Here's how the part is built. I have some questions about the finished solid (model axes, mm). Round coordinates to 2 decimals unless told otherwise and drop trailing zeros. Order: outer loops, then holes, each group sorted by start corner. A loop starts at its lowest first (then second) coordinate and runs counter-clockwise, first axis right, second up. Notation, with made-up numbers: (-5, 31) - (29, 31) arc R28 cw to (29, 67) - close; hole circle Ø10 at (75, -23). An arc over 180 degrees is marked (long way). One line per item, written item: value.
from build123d import *

# Parameters (mm, degrees)
F1_DEPTH = 85
F2_W     = 3.5
F2_H     = 3.5
F3_DEPTH = 3.5
F4_W     = 3.5
F4_H     = 3.5
F5_DEPTH = 3.5


with BuildPart() as f1:
    # F0 (on Top) → F1 (new body)
    with BuildSketch(Plane.XY):
        Polygon((-25, -42.409548), (-25, -34.409548), (-32.608452, -36.881684), (-30.81234, -42.409548), align=None)
    extrude(amount=F1_DEPTH)

    # F2 (on face) → F3 (cut)
    with BuildSketch(Plane.YZ.offset(-25)):
        with Locations((-37.659548, 6.25)):
            Rectangle(F2_W, F2_H)
        with Locations((-37.659548, 28.25)):
            Rectangle(F2_W, F2_H)
    extrude(amount=-F3_DEPTH, mode=Mode.SUBTRACT)

    # F4 (on face) → F5 (cut)
    with BuildSketch(Plane(origin=(7.725425, -23.776413, 0), x_dir=(-0.951057, -0.309017, 0), z_dir=(-0.309017, 0.951057, 0))):
        with Locations((37.659548, 6.25)):
            Rectangle(F4_W, F4_H)
        with Locations((37.659548, 28.25)):
            Rectangle(F4_W, F4_H)
    extrude(amount=-F5_DEPTH, mode=Mode.SUBTRACT)


solid = f1.part
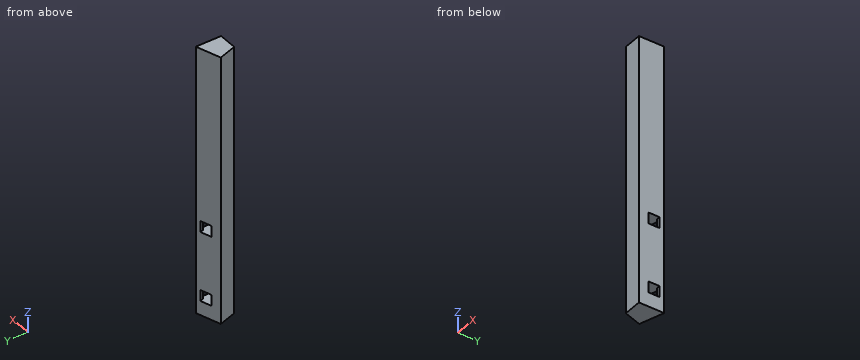
Q1. If I drill on line 1 along Z through (x, y) = (-27.75, -36.5); line 2 along Y through (x, z) = (-25.5, 72); line 3 along Y through (x, z) = (-26, 38.5), over which ranges is the centre line in solid material (lowest first)?
Results list:
line 1: 0 to 4.5, 8 to 26.5, 30 to 85
line 2: -42.41 to -34.57
line 3: -42.41 to -34.73
Q2. Will these pins go through, and if not, where does the flat tip stop? pin 1 (1 mm diameter, centred on x = -26.5, z = 28, fed in from +Y); pin 2 (2 mm diameter, centred on y = -38.5, z = 29.5, fed in from -X); pin 3 (1.5 mm diameter, centred on x = -29, z = 19, fed in from +Y).
Results list:
pin 1: y = -34.73
pin 2: x = -32.41
pin 3: y = -35.47
Q3. If we section it at A-A, the plane y = -38.5: Please give me the cut outline in (x, z).
Results list:
outline: (-32.08, 0) - (-25, 0) - (-25, 4.5) - (-28.93, 4.5) - (-28.93, 8) - (-25, 8) - (-25, 26.5) - (-28.93, 26.5) - (-28.93, 30) - (-25, 30) - (-25, 85) - (-32.08, 85) - close
Q4. If we section it at C-C, the plane x = -31.75: Please give me the cut outline in (y, z).
Results list:
outline: (-39.52, 0) - (-36.6, 0) - (-36.6, 85) - (-39.52, 85) - close
Q5. If we section it at B-B, the plane z = 69.5: Please give me the cut outline in (x, y).
Results list:
outline: (-32.61, -36.88) - (-30.81, -42.41) - (-25, -42.41) - (-25, -34.41) - close
